```python
from build123d import *

# Parameters (mm, degrees)
SKETCH1_W                        = 15
SKETCH1_H                        = 6
MAIN_BODY_EXT_DEPTH              = 8.3
EMISSION_PATH_EXT_DEPTH          = 9
SKETCH3_R                        = 1.25
EMISSION_AND_GRIN_CUT_DEPTH      = 20.092931
SKETCH4_R                        = 1
DRUM_LENS_CUT_DEPTH              = 13
SKETCH41_R                       = 1
ADDTL_LIGHT_SOURCE_DEPTH         = 5
SKETCH5_W                        = 15
SKETCH5_H                        = 7.3
FILTERSET_CUT1_DEPTH             = 1
FILTERSET_CUT2_DEPTH             = 4
SKETCH10_R                       = 2.5
EMISSION_LENS_CUT_DEPTH          = 8.5
SKETCH15_R                       = 0.795
MAGNETS_CUT_DEPTH                = 0.9
SCREW_HOLES_CUT_DEPTH            = 20.507434
SCREW_HOLES_CUT_DEPTH_BACK       = 3
SKETCH18_R                       = 0.375
EXTERNAL_FILLET_1_R              = 1.5
CUT_EXTRUDE8_DEPTH               = 14.011149
CUT_EXTRUDE8_DEPTH_BACK          = 4
SKETCH28_R                       = 1.5
CUT_EXTRUDE9_DEPTH               = 3
CUT_EXTRUDE_ORIGINAL_LIGHT_DEPTH = 0.7
CUT_EXTRUDE_ADDTL_LIGHT_DEPTH    = 0.7
SKETCH29_R                       = 0.375
CUT_EXTRUDE11_DEPTH              = 2.5
SKETCH32_W                       = 2
SKETCH32_H                       = 2.36
CUT_EXTRUDE14_DEPTH              = 0.7
SKETCH45_W                       = 2.36
SKETCH45_H                       = 2
CUT_EXTRUDE19_DEPTH              = 0.7
CUT_EXTRUDE16_DEPTH              = 9
CUT_EXTRUDE17_REACH              = 13.945
SKETCH37_R                       = 2


with BuildPart() as part:
    # Sketch1 → Main Body Ext (new body)
    with BuildSketch(Plane(origin=(0, 0, 0), x_dir=(1, 0, 0), z_dir=(0, 1, 0))):
        Rectangle(SKETCH1_W, SKETCH1_H)
    extrude(amount=MAIN_BODY_EXT_DEPTH)

    # Sketch8 → Emission Path Ext (add)
    with BuildSketch(Plane(origin=(0, 8.3, 0), x_dir=(1, 0, 0), z_dir=(0, 1, 0))):
        Polygon((-2.75, 3), (-1.5, 1.75), (-1.5, -3), (-7.5, -3), (-7.5, 3), align=None)
    extrude(amount=EMISSION_PATH_EXT_DEPTH)

    # Sketch3 → Emission and Grin Cut (cut, through all)
    with BuildSketch(Plane.XZ):
        with Locations(Location((-4.5, 0, 0), (0, 0, 270))):
            Circle(SKETCH3_R)
    extrude(amount=-EMISSION_AND_GRIN_CUT_DEPTH, mode=Mode.SUBTRACT)

    # Sketch4 → Drum Lens Cut (cut)
    with BuildSketch(Plane(origin=(7.5, 0, 0), x_dir=(0, 0, -1), z_dir=(1, 0, 0))):
        with Locations((0, 3)):
            Circle(SKETCH4_R)
    extrude(amount=-DRUM_LENS_CUT_DEPTH, mode=Mode.SUBTRACT)

    # Sketch41 → Addtl Light Source (cut)
    with BuildSketch(Plane(origin=(0, 8.3, 0), x_dir=(1, 0, 0), z_dir=(0, 1, 0))):
        with Locations(Location((1.5, 0, 0), (0, 0, 270))):
            Circle(SKETCH41_R)
    extrude(amount=-ADDTL_LIGHT_SOURCE_DEPTH, mode=Mode.SUBTRACT)

    # Sketch5 → FilterSet Cut1 (cut)
    with BuildSketch(Plane.XY.offset(3)):
        with Locations((0, 4.65)):
            Rectangle(SKETCH5_W, SKETCH5_H)
    extrude(amount=-FILTERSET_CUT1_DEPTH, mode=Mode.SUBTRACT)

    # Sketch6 → FilterSet Cut2 (cut)
    with BuildSketch(Plane.XY.offset(2)):
        with BuildLine():
            Line((5.3, 4.5), (5.3, 1.8))
            ThreePointArc((5.3, 1.8), (5.7, 1.4), (5.3, 1))
            Line((5.3, 1), (4.1, 1))
            ThreePointArc((4.1, 1), (3.7, 1.4), (4.1, 1.8))
            Line((4.1, 1.8), (4.1, 4.5))
            ThreePointArc((4.1, 4.5), (4.7, 5.1), (5.3, 4.5))
        make_face()
        with BuildLine():
            Line((-6.9, 7.9), (-6.9, 7.5))
            ThreePointArc((-6.9, 7.5), (-6.782843, 7.217157), (-6.5, 7.1))
            Line((-6.5, 7.1), (-2.5, 7.1))
            ThreePointArc((-2.5, 7.1), (-2.217157, 7.217157), (-2.1, 7.5))
            Line((-2.1, 7.5), (-2.1, 7.9))
            ThreePointArc((-2.1, 7.9), (-2.217157, 8.182843), (-2.5, 8.3))
            Line((-2.5, 8.3), (-6.5, 8.3))
            ThreePointArc((-6.5, 8.3), (-6.782843, 8.182843), (-6.9, 7.9))
        make_face()
        with BuildLine():
            Line((-2.605887, 6.591169), (-6.848528, 2.348528))
            ThreePointArc((-6.848528, 2.348528), (-6.848528, 1.5), (-6, 1.5))
            Line((-6, 1.5), (-1.757359, 5.742641))
            ThreePointArc((-1.757359, 5.742641), (-1.757359, 6.591169), (-2.605887, 6.591169))
        make_face()
        with BuildLine():
            Line((3.112092, 6.591169), (-1.130548, 2.348528))
            ThreePointArc((-1.130548, 2.348528), (-1.130548, 1.5), (-0.28202, 1.5))
            Line((-0.28202, 1.5), (3.96062, 5.742641))
            ThreePointArc((3.96062, 5.742641), (3.96062, 6.591169), (3.112092, 6.591169))
        make_face()
    extrude(amount=-FILTERSET_CUT2_DEPTH, mode=Mode.SUBTRACT)

    # Sketch10 → Emission Lens Cut (cut)
    with BuildSketch(Plane(origin=(0, 17.3, 0), x_dir=(1, 0, 0), z_dir=(0, 1, 0))):
        with Locations(Location((-4.5, 0, 0), (0, 0, 270))):
            Circle(SKETCH10_R)
    extrude(amount=-EMISSION_LENS_CUT_DEPTH, mode=Mode.SUBTRACT)

    # Sketch15 → Magnets Cut (cut)
    with BuildSketch(Plane.XZ):
        with Locations(Location((-6.25, -1.875, 0), (0, 0, 270))):
            Circle(SKETCH15_R)
        with Locations(Location((-6.25, 1.875, 0), (0, 0, 270))):
            Circle(SKETCH15_R)
        with Locations(Location((2.5, 0, 0), (0, 0, 270))):
            Circle(SKETCH15_R)
    extrude(amount=-MAGNETS_CUT_DEPTH, mode=Mode.SUBTRACT)

    # Sketch18 → Screw Holes Cut (cut, two sides: drawn at the far end of the back side and taken through both)
    with BuildSketch(Plane.XY.offset(2).offset(-SCREW_HOLES_CUT_DEPTH_BACK)):
        with Locations(Location((-6.5, 4, 0), (0, 0, 180))):
            Circle(SKETCH18_R)
        with Locations(Location((5.5, 6.5, 0), (0, 0, 180))):
            Circle(SKETCH18_R)
        with Locations((0.25, 1)):
            Circle(SKETCH18_R)
    extrude(amount=SCREW_HOLES_CUT_DEPTH + SCREW_HOLES_CUT_DEPTH_BACK, mode=Mode.SUBTRACT)

    # External Fillet 1
    # the kernel refuses this fillet: 1.5 mm, written as the material it takes off along each edge
    with BuildSketch(Plane(origin=(-7.5, -3.75, -3), x_dir=(1, 0, 0), z_dir=(0, 1, 0))) as external_fillet_1_piece_1:
        with BuildLine():
            CenterArc((EXTERNAL_FILLET_1_R, -EXTERNAL_FILLET_1_R), EXTERNAL_FILLET_1_R, 90, 90)
            Line((0, -EXTERNAL_FILLET_1_R), (0, 0))
            Line((0, 0), (EXTERNAL_FILLET_1_R, 0))
        make_face()
    extrude(amount=24.8, mode=Mode.SUBTRACT)
    with BuildSketch(Plane(origin=(-1.5, 8.3, 3), x_dir=(0, 0, -1), z_dir=(0, 1, 0))) as external_fillet_1_piece_2:
        with BuildLine():
            CenterArc((EXTERNAL_FILLET_1_R, EXTERNAL_FILLET_1_R), EXTERNAL_FILLET_1_R, 180, 90)
            Line((0, EXTERNAL_FILLET_1_R), (0, 0))
            Line((0, 0), (EXTERNAL_FILLET_1_R, 0))
        make_face()
    extrude(amount=12.75, mode=Mode.SUBTRACT)

    # Sketch28 → Cut-Extrude8 (cut, two sides: drawn at the far end of the back side and taken through both)
    with BuildSketch(Plane(origin=(0, 7.1, 0), x_dir=(1, 0, 0), z_dir=(0, 1, 0)).offset(-CUT_EXTRUDE8_DEPTH_BACK)):
        with Locations(Location((-4.5, 0, 0), (0, 0, 180))):
            Circle(SKETCH28_R)
    extrude(amount=CUT_EXTRUDE8_DEPTH + CUT_EXTRUDE8_DEPTH_BACK, mode=Mode.SUBTRACT)

    # Sketch14 → Cut-Extrude9 (cut)
    with BuildSketch(Plane.XZ):
        Polygon((7.5, -3), (7.5, -1.891585), (7.056634, -3), align=None)
    extrude(amount=-CUT_EXTRUDE9_DEPTH, mode=Mode.SUBTRACT)

    # Sketch12 → Cut-Extrude Original Light (cut)
    with BuildSketch(Plane(origin=(7.5, 0, 0), x_dir=(0, 0, -1), z_dir=(1, 0, 0))):
        with BuildLine():
            Line((1.6, 5.94), (-1.6, 5.94))
            Line((-1.6, 5.94), (-2, 5.94))
            Line((-2, 5.94), (-2, 1.33))
            Line((-2, 1.33), (1.6, 1.33))
            ThreePointArc((1.6, 1.33), (1.882843, 1.447157), (2, 1.73))
            Line((2, 1.73), (2, 5.54))
            ThreePointArc((2, 5.54), (1.882843, 5.822843), (1.6, 5.94))
        make_face()
    extrude(amount=-CUT_EXTRUDE_ORIGINAL_LIGHT_DEPTH, mode=Mode.SUBTRACT)

    # Sketch44 → Cut-Extrude Addtl Light (cut)
    with BuildSketch(Plane(origin=(0, 8.3, 0), x_dir=(1, 0, 0), z_dir=(0, 1, 0))):
        with BuildLine():
            Line((-0.17, -2), (4.44, -2))
            Line((4.44, -2), (4.44, 1.6))
            ThreePointArc((4.44, 1.6), (4.322843, 1.882843), (4.04, 2))
            Line((4.04, 2), (0.23, 2))
            ThreePointArc((0.23, 2), (-0.052843, 1.882843), (-0.17, 1.6))
            Line((-0.17, 1.6), (-0.17, -2))
        make_face()
    extrude(amount=-CUT_EXTRUDE_ADDTL_LIGHT_DEPTH, mode=Mode.SUBTRACT)

    # Sketch29 → Cut-Extrude11 (cut)
    with BuildSketch(Plane(origin=(7.5, 0, 0), x_dir=(0, 0, -1), z_dir=(1, 0, 0))):
        with Locations((2, 6.5)):
            Circle(SKETCH29_R)
    extrude(amount=-CUT_EXTRUDE11_DEPTH, mode=Mode.SUBTRACT)

    # Sketch32 → Cut-Extrude14 (cut)
    with BuildSketch(Plane(origin=(7.5, 0, 0), x_dir=(0, 0, -1), z_dir=(1, 0, 0))):
        with Locations((0, 7.12)):
            Rectangle(SKETCH32_W, SKETCH32_H)
    extrude(amount=-CUT_EXTRUDE14_DEPTH, mode=Mode.SUBTRACT)

    # Sketch45 → Cut-Extrude19 (cut)
    with BuildSketch(Plane(origin=(0, 8.3, 0), x_dir=(1, 0, 0), z_dir=(0, 1, 0))):
        with Locations((5.62, 0)):
            Rectangle(SKETCH45_W, SKETCH45_H)
    extrude(amount=-CUT_EXTRUDE19_DEPTH, mode=Mode.SUBTRACT)

    # Sketch33 → Cut-Revolve1 (revolve, cut)
    with BuildSketch(Plane.XY, mode=Mode.PRIVATE) as cut_revolve1_sk:
        with BuildLine():
            Line((6.8, 3), (5.3, 3))
            ThreePointArc((5.3, 3), (5.73934, 4.06066), (6.8, 4.5))
            Line((6.8, 4.5), (6.8, 3))
        make_face()
    revolve(cut_revolve1_sk.sketch.rotate(Axis((6.8, 3, 0), (-1, 0, 0)), 84.26086), axis=Axis((6.8, 3, 0), (-1, 0, 0)), mode=Mode.SUBTRACT)

    # Sketch47 → Cut-Revolve2 (revolve, cut)
    with BuildSketch(Plane(origin=(1.5, 0, 0), x_dir=(0, 0, -1), z_dir=(1, 0, 0))):
        with BuildLine():
            Line((-1.5, 7.6), (0, 7.6))
            Line((0, 7.6), (0, 6.137287))
            ThreePointArc((0, 6.137287), (-1.04756, 6.563498), (-1.5, 7.6))
        make_face()
    revolve(axis=Axis((1.5, 7.6, 0), (0, -1, 0)), mode=Mode.SUBTRACT)

    # Sketch36 → Cut-Extrude16 (cut)
    with BuildSketch(Plane(origin=(0, 17.3, 0), x_dir=(1, 0, 0), z_dir=(0, 1, 0))):
        with BuildLine():
            Line((-7.5, -1.5), (-7.5, -3))
            Line((-7.5, -3), (-6, -3))
            ThreePointArc((-6, -3), (-7.06066, -2.56066), (-7.5, -1.5))
        make_face()
    extrude(amount=-CUT_EXTRUDE16_DEPTH, mode=Mode.SUBTRACT)

    # Sketch37 → Cut-Extrude17 (cut, up to next)
    with BuildSketch(Plane(origin=(0, 8.8, 0), x_dir=(1, 0, 0), z_dir=(0, 1, 0)), mode=Mode.PRIVATE) as cut_extrude17_sk1:
        with Locations(Location((-4.5, 0, 0), (0, 0, 180))):
            Circle(SKETCH37_R)
    cut_extrude17_tool1 = extrude(cut_extrude17_sk1.sketch, amount=-CUT_EXTRUDE17_REACH, mode=Mode.PRIVATE) & part.part
    add(cut_extrude17_tool1.solids().sort_by_distance((-4.5, 8.8, 0))[0], mode=Mode.SUBTRACT)


solid = part.part
```
Work out the finished part from the listing and answer in its coordinate system (mm). A direction names the side the tool comes from. Give positions to 0.01 mm unless a question says otherwise; leave off trailing zeros. One line per item, written item: value. Start each with the question number.
1. Section A-A, the plane x = -4.75 is taken. Count the separate pieces of the cut face and the enclosed holes in it, then the cut area to 3 significant figures.
2. Which of the six approach directions +Z, -Z, +X, -X, +Y, -Y give full straight-line access (tool end or side, diameter ignored) to faces 5 (the face through (3, 2, 0)), 6 (the face through (5, 3, -2)), 7 (the face through (3, 0.9, 0))?
3. For a pull along X with two mould halves and no side action, classify faces 1 (the face through (-1.14, 1.51, 0.03)), 2 (the face through (6, 8, -1)), 3 (the face through (7.5, 7.1, 1.5)), 4 (the face through (0.55, 4.03, 0.92)) as released by +X, released by -X, zero draft, split by the parting line, or undercut.
4. Each of these flat-tipped pins is pushed along its axis until it touches: pin 1 Ø0.8 at (x, z) = (7, 0.5) entering from +Y; pin 2 Ø0.5 at (x, z) = (2.5, 0) entering from -Y; pin 3 Ø3.5 at (y, z) = (13.5, -1) entering from +X. Where does it stop, or does it pass through?
5. Consider line 1 (Y direction, x = -5.5, z = 1.95); line 2 (Y direction, x = -6, z = 1.4); line 3 (X direction, y = 11.5, z = -0.1). Determine where each line is inside the solid, lowest interval first.
Filled sheet:
1. separate pieces: 4
1. enclosed holes: 0
1. area: 26.1 mm²
2. face 5: +X
2. face 6: +Z
2. face 7: -Y
3. face 1: undercut
3. face 2: zero draft
3. face 3: released by +X
3. face 4: undercut
4. pin 1: y = 7.6
4. pin 2: y = 0.9
4. pin 3: x = -1.5
5. line 1: 0.9 to 2, 3.7 to 7.1, 8.3 to 8.8
5. line 2: 0.9 to 1.5, 3.2 to 7.1, 8.3 to 8.8
5. line 3: -7.5 to -7, -2 to -1.5
